```python
from build123d import *

# Parameters (mm, degrees)
F1_W        = 68.6
F1_H        = 53.3
F1_R        = 1.5
F2_DEPTH    = 2.4
F4_DEPTH    = 39
F6_DEPTH    = 69.6
F7_T1_DEPTH = 69.6
F8_W        = 29.3
F8_H        = 14
F9_DEPTH    = 25.4
F10_W       = 26
F10_H       = 14
F11_DEPTH   = 25.4


# Not quite as in the source:
# - a fillet or chamfer that OpenCascade refuses, or shapes differently, is made with other operations: its cross-section is extruded or revolved along the edge and cut away or added


with BuildPart() as f2:
    # F1 (on Top) → F2 (new body)
    with BuildSketch(Plane.XY):
        Polygon((-68.6, 0), (-68.6, 53.3), (0, 53.3), (0, 56.3), (-71.6, 56.3), (-71.6, -3), (0, -3), (0, 0), align=None)
        with Locations((-34.3, 26.65)):
            Rectangle(F1_W, F1_H)
        with Locations((-66.4, 7.9)):
            Circle(F1_R, mode=Mode.SUBTRACT)
        with Locations((-15.2, 2.2)):
            Circle(F1_R, mode=Mode.SUBTRACT)
        with Locations((-66.3, 35.8)):
            Circle(F1_R, mode=Mode.SUBTRACT)
        with Locations((-13.9, 51.1)):
            Circle(F1_R, mode=Mode.SUBTRACT)
    extrude(amount=F2_DEPTH)

    # F3 (on face) → F4 (join)
    with BuildSketch(Plane.XY.offset(2.4)):
        Polygon((0, 54.3), (0, 56.3), (-71.6, 56.3), (-71.6, -3), (0, -3), (0, -1), (-69.6, -1), (-69.6, 54.3), align=None)
    extrude(amount=F4_DEPTH)

    # F5 (on face) → F6 (join, through all)
    with BuildSketch(Plane.YZ.offset(-69.6)):
        Polygon((2, 41.4), (-1, 41.4), (-2.3718131706, 41.4), (-2.3718131706, 32.4), (-1, 32.4), (2, 32.4), (2, 35.4), (-1, 35.4), (-1, 38.4), (2, 38.4), align=None)
        Polygon((55.6718131706, 32.4), (55.6718131706, 41.4), (54.3, 41.4), (51.3, 41.4), (51.3, 38.4), (54.3, 38.4), (54.3, 35.4), (51.3, 35.4), (51.3, 32.4), (54.3, 32.4), align=None)
    extrude(amount=F6_DEPTH)

    # F7: fillet of radius 3 on 2 edges, made by hand

    # F7_s2 → F7_t1 (join)
    with BuildSketch(Plane.YZ.offset(-69.6)):
        with BuildLine():
            add(Edge.make_bspline(
                [(2, 32.4), (-1, 32.4), (-1, 29.4)],
                knots=[0, 0, 0, 1, 1, 1], degree=2, weights=[1, 1, 1]))
            Line((-1, 29.4), (-1, 32.4))
            Line((-1, 32.4), (2, 32.4))
        make_face()
        with BuildLine():
            add(Edge.make_bspline(
                [(54.3, 29.4), (54.3, 32.4), (51.3, 32.4)],
                knots=[0, 0, 0, 1, 1, 1], degree=2, weights=[1, 1, 1]))
            Line((51.3, 32.4), (54.3, 32.4))
            Line((54.3, 32.4), (54.3, 29.4))
        make_face()
    extrude(amount=F7_T1_DEPTH)

    # F8 (on face) → F9 (cut)
    with BuildSketch(Plane.YZ.offset(-69.6)):
        with Locations((27.65, 24.4)):
            Rectangle(F8_W, F8_H)
    extrude(amount=-F9_DEPTH, mode=Mode.SUBTRACT)

    # F10 (on face) → F11 (cut)
    with BuildSketch(Plane(origin=(0, 56.3, 0), x_dir=(-1, 0, 0), z_dir=(0, 1, 0))):
        with Locations((13, 24.4)):
            Rectangle(F10_W, F10_H)
    extrude(amount=-F11_DEPTH, mode=Mode.SUBTRACT)


solid = f2.part
```
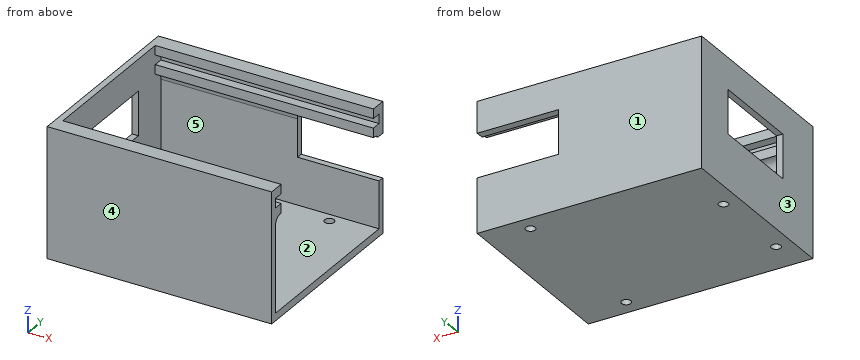
Can you work these out from the model? Positions are in its coordinate system, mm. Face numbers are marked on the shaded views. A direction names the side the tool comes from. Round coordinates to 2 decimals unless told otherwise and drop trailing zeros. Order: outer loops, then holes, each group sorted by start corner. A loop starts at its lowest first (then second) coordinate and runs counter-clockwise, first axis right, second up. Notation, with made-up numbers: (68.5, 76) -> (127.5, 76) arc R17 ccw to (127.5, 92) -> close; hole circle Ø1 at (33.25, 43.5). An arc over 180 degrees is marked (long way). Return JSON: item names as keys, results as strings. Group by question number.
1. I need wall thicknesses on line 1 (Y direction, x = -10, z = 35); line 2 (Y direction, x = -41, z = 26.5); line 3 (X direction, y = 2, z = 1). Which ranges of each line are inside material? Lowest first, please. Write a range as [from, to].
2. If we section it at D-D, the plane x = -66.3: Count the separate pieces of the cut face and the enclosed holes in it, then the cut area to 3 significant figures.
3. If we section it at A-A, the plane z = 19.5: Write out the boundary of the cut face in (x, y), then the cut area to 3 significant figures.
4. If we section it at B-B, the plane y = 38.5: Write out the boundary of the cut face in (x, z), then the cut area to 3 significant figures.
5. If we section it at C-C, the plane y = 7.9: Write out the boundary of the cut face in (x, z).
6. Will these pins go through, and if not, where does the flat tip stop? pin 1 (1 mm diameter, centred on y = 41, z = 5, fed in from +X); pin 2 (1 mm diameter, centred on x = -23, z = 19.5, fed in from +Y); pin 3 (0.8 mm diameter, centred on y = 54.5, z = 25.5, fed in from +X); pin 4 (6 mm diameter, centred on y = 17, z = 20.5, fed in from +X).
7. We'd pull the mould along Y, two halves only. Please class the marked faces 1, 2 and 3: released by +Y, released by -Y, zero draft, split by the parting line, or undercut.
8. Which directions (+Z, -Z, +X, -X, +Y, -Y) give clear straight access to the entire face, cutting with the end or side of a thin tool? Please do the marked faces 4 and 5.
Output values:
{
 "1": {"line 1": "[-3, 2], [51.3, 56.3]", "line 2": "[-3, -1], [54.3, 56.3]", "line 3": "[-71.6, -16.69], [-13.71, 0]"},
 "2": {"separate pieces": "3", "enclosed holes": "0", "area": "323 mm²"},
 "3": {"outline": "(-71.6, -3) -> (0, -3) -> (0, -1) -> (-69.6, -1) -> (-69.6, 13) -> (-71.6, 13) -> close; (-71.6, 42.3) -> (-69.6, 42.3) -> (-69.6, 54.3) -> (-26, 54.3) -> (-26, 56.3) -> (-71.6, 56.3) -> close", "area": "286 mm²"},
 "4": {"outline": "(-71.6, 0) -> (0, 0) -> (0, 2.4) -> (-69.6, 2.4) -> (-69.6, 17.4) -> (-71.6, 17.4) -> close; (-71.6, 31.4) -> (-69.6, 31.4) -> (-69.6, 41.4) -> (-71.6, 41.4) -> close", "area": "222 mm²"},
 "5": {"outline": "(-71.6, 0) -> (-67.9, 0) -> (-67.9, 2.4) -> (-69.6, 2.4) -> (-69.6, 41.4) -> (-71.6, 41.4) -> close; (-64.9, 0) -> (0, 0) -> (0, 2.4) -> (-64.9, 2.4) -> close"},
 "6": {"pin 1": "x = -69.6", "pin 2": "y = -1", "pin 3": "x = -26", "pin 4": "through"},
 "7": {"face 1": "released by +Y", "face 2": "undercut", "face 3": "zero draft"},
 "8": {"face 4": "+Z, -Z, +X, -X, -Y", "face 5": "+X"}
}
